```python
from build123d import *

# Parameters (mm, degrees)
EXTRUDE_1_DEPTH = 5
FILLET_1_R      = 1.4
CHAMFER_1_SIZE  = 0.4


with BuildPart() as part:
    # 草图1 → 凸台-拉伸1 (new body)
    with BuildSketch(Plane(origin=(0, 0, 0), x_dir=(1, 0, 0), z_dir=(0, 1, 0))):
        with BuildLine():
            Line((-0.1, 30), (-2.6, 30))
            Line((-2.6, 30), (-2.6, 11.714947716))
            ThreePointArc((-2.6, 11.714947716), (0.102243606, -11.999564419), (2.4, 11.757550765))
            Line((2.4, 11.757550765), (2.4, 30))
            Line((2.4, 30), (-0.1, 30))
        make_face()
    extrude(amount=EXTRUDE_1_DEPTH)

    # 圆角1
    fillet_1_edges = [part.edges().sort_by_distance(p)[0] for p in [
        (-2.6, 2.5, -11.714947716),
        (2.4, 2.5, -11.757550765),
    ]]
    fillet(fillet_1_edges, radius=FILLET_1_R)

    # 倒角1
    chamfer_1_edges = [part.edges().sort_by_distance(p)[0] for p in [
        (-0.1, 5, -30),
        (2.4, 0, -21.424951362),
        (2.4, 5, -21.424951362),
        (0.093604691, 0, 11.999634918),
        (0.093604691, 5, 11.999634918),
        (-2.6, 5, -21.394528911),
        (2.678433931, 0, -12.011994881),
        (2.678433931, 5, -12.011994881),
        (-2.871932044, 0, -11.959924127),
        (-2.871932044, 5, -11.959924127),
        (-2.6, 0, -21.394528911),
        (-0.1, 0, -30),
        (-2.6, 2.5, -30),
        (2.4, 2.5, -30),
    ]]
    chamfer(chamfer_1_edges, length=CHAMFER_1_SIZE)


solid = part.part
```
For this review, take the finished solid that the model builds, in its own axes (mm). A direction names the side the tool comes from. Round coordinates to 2 decimals unless told otherwise and drop trailing zeros. Write each loop counter-clockwise with the first axis right and the second up, starting at its lowest first coordinate (ties: lowest second). Pieces come first, ordered by that corner, then holes. Notation, with made-up numbers: (-3.75, 16) - (30.25, 16) arc R32 ccw to (30.25, 45) - close; hole circle Ø6 at (23.25, 51). An arc over 180 degrees is marked (long way). Answer as a JSON object with one key per item and string values.
1. We need section A-A on z = -20.5. Give the boundary of the cut face in (x, y).
Response values:
{"outline": "(-2.6, 0.4) - (-2.2, 0) - (2, 0) - (2.4, 0.4) - (2.4, 4.6) - (2, 5) - (-2.2, 5) - (-2.6, 4.6) - close"}
2. To check wall thickness, follow line 1 along X through (y, z) = (3.85, -27.5); line 2 along Z through (x, y) = (-0.25, 2.1); line 3 along Z through (x, y) = (-7.75, 2.35). State the ranges of each line that lie inside material, in increasing order.
Response values:
{"line 1": "x = -2.6 to 2.4", "line 2": "z = -30 to 12", "line 3": "z = -9.16 to 9.16"}
3. For pin 1 Ø3 at (y, z) = (3, 2) entering from -X, flat-tipped, find the tip position at first contact; note if it passes through.
Response values:
{"pin 1": "stops at x = -11.99"}
4. Draft analysis for pull direction Z (two halves, no side actions). For faces 3 (the face through (0, 2, 12)), 4 (the face through (-2.865, 2.529, -11.97)), 5 (the face through (2.4, 2, -21)), state which applies: +Z half, -Z half, draft (parallel to the pull), parting line (faces both ways), or undercut.
Response values:
{"face 3": "parting line", "face 4": "-Z half", "face 5": "draft"}
5. Tool access review of faces 1 (the face through (0, 2, -30)), 2 (the face through (-2.6, 2, -21)): name each direction out of +Z, -Z, +X, -X, +Y, -Y from which nothing blocks a thin tool from reaching the whole face with its end or side.
Response values:
{"face 1": "-Z, +X, -X, +Y, -Y", "face 2": "-Z, -X, +Y, -Y"}
6. We need section B-B on y = 3.35. Give the boundary of the cut face in (x, z).
Response values:
{"outline": "(-3.58, -11.45) arc R1.4 cw to (-2.6, -12.79) - (-2.6, -29.6) - (-2.2, -30) - (2, -30) - (2.4, -29.6) - (2.4, -12.85) arc R1.4 cw to (3.4, -11.51) arc R12 ccw (long way) to start"}
